Source: CAD feature listing. Evaluate the final solid. Frame: model axes, mm. A direction names the side the tool comes from. Give positions to 0.01 mm unless a question says otherwise; leave off trailing zeros. Loops run counter-clockwise (first coordinate to the right, second up) from the corner with the lowest first, then second, coordinate; pieces in that order, holes last.
```python
from build123d import *

# Parameters (mm, degrees)
F0_W     = 78
F0_H     = 157.7
F0_W_2   = 73.4
F0_H_2   = 153.1
F0_R     = 2
F0_R_2   = 2.5
F1_DEPTH = 2.3
F2_DEPTH = 9
F3_DEPTH = 7.5
F4_DEPTH = 25
F5_R     = 12
F6_R     = 14


with BuildPart() as f1:
    # F0 (on Front) → F1 (new body)
    with BuildSketch(Plane.XZ):
        Rectangle(F0_W, F0_H)
        Rectangle(F0_W_2, F0_H_2, mode=Mode.SUBTRACT)
        Rectangle(F0_W_2, F0_H_2)
        with Locations((-31.5, -22.85)):
            Circle(F0_R, mode=Mode.SUBTRACT)
        Polygon((-20, -22.85), (0, -9.85), (20, -22.85), (0, -35.85), align=None, mode=Mode.SUBTRACT)
        with Locations((31.5, -22.85)):
            Circle(F0_R, mode=Mode.SUBTRACT)
        with Locations((-30.7, 36.55)):
            Circle(F0_R, mode=Mode.SUBTRACT)
        with BuildLine():
            add(Edge.make_bspline(
                [(-20.35, 36.55), (-20.35, 29.1887840678), (-10.375, 32.8693920339), (-0.4, 36.55), (-10.375, 40.2306079661), (-20.35, 43.9112159322), (-20.35, 36.55)],
                knots=[0, 0, 0, 2.0943951024, 2.0943951024, 4.1887902048, 4.1887902048, 6.2831853072, 6.2831853072, 6.2831853072], degree=2, weights=[1, 0.5, 1, 0.5, 1, 0.5, 1]))
        make_face(mode=Mode.SUBTRACT)
        with Locations((-20.5, 60.55)):
            Circle(F0_R_2, mode=Mode.SUBTRACT)
        with BuildLine():
            ThreePointArc((2.8259154066, 10.0287804232), (1.4142570551, 10.119681178), (0, 10.15))
            ThreePointArc((0, 10.15), (-1.4142571139, 10.1196811755), (-2.825915524, 10.0287804131))
            ThreePointArc((-2.825915524, 10.0287804131), (-5.6846492436, 9.656687973), (-8.5, 9.036517527))
            Line((-8.5, 9.036517527), (0, 26.15))
            Line((0, 26.15), (8.5, 9.036517527))
            ThreePointArc((8.5, 9.036517527), (5.6846491856, 9.6566879832), (2.8259154066, 10.0287804232))
        make_face(mode=Mode.SUBTRACT)
        with BuildLine():
            add(Edge.make_bspline(
                [(20.35, 36.55), (20.35, 43.9112159322), (10.375, 40.2306079661), (0.4, 36.55), (10.375, 32.8693920339), (20.35, 29.1887840678), (20.35, 36.55)],
                knots=[0, 0, 0, 2.0943951024, 2.0943951024, 4.1887902048, 4.1887902048, 6.2831853072, 6.2831853072, 6.2831853072], degree=2, weights=[1, 0.5, 1, 0.5, 1, 0.5, 1]))
        make_face(mode=Mode.SUBTRACT)
        with Locations((30.7, 36.55)):
            Circle(F0_R, mode=Mode.SUBTRACT)
        with Locations((0, 72.05)):
            Circle(F0_R, mode=Mode.SUBTRACT)
        with Locations((20.5, 60.55)):
            Circle(F0_R_2, mode=Mode.SUBTRACT)
        Polygon((20, -22.85), (0, -9.85), (-20, -22.85), (0, -35.85), align=None)
        with BuildLine():
            ThreePointArc((-2.825915524, 10.0287804131), (-1.4142571139, 10.1196811755), (0, 10.15))
            ThreePointArc((0, 10.15), (1.4142570551, 10.119681178), (2.8259154066, 10.0287804232))
            ThreePointArc((2.8259154066, 10.0287804232), (5.6846491856, 9.6566879832), (8.5, 9.036517527))
            Line((8.5, 9.036517527), (0, 26.15))
            Line((0, 26.15), (-8.5, 9.036517527))
            ThreePointArc((-8.5, 9.036517527), (-5.6846492436, 9.656687973), (-2.825915524, 10.0287804131))
        make_face()
        with BuildLine():
            ThreePointArc((-0.54, 12.5195971139), (-1.1980972895, 10.8292141972), (-2.825915524, 10.0287804131))
            ThreePointArc((-2.825915524, 10.0287804131), (-4.8819027105, 14.2099800306), (-0.54, 12.5195971139))
        make_face(mode=Mode.SUBTRACT)
        with BuildLine():
            ThreePointArc((5.54, 12.5195971139), (4.7303828733, 10.6776943636), (2.8259154066, 10.0287804232))
            ThreePointArc((2.8259154066, 10.0287804232), (1.3496171267, 14.3614998642), (5.54, 12.5195971139))
        make_face(mode=Mode.SUBTRACT)
        with BuildLine():
            add(Edge.make_bspline(
                [(-20.35, 36.55), (-20.35, 29.1887840678), (-10.375, 32.8693920339), (-0.4, 36.55), (-10.375, 40.2306079661), (-20.35, 43.9112159322), (-20.35, 36.55)],
                knots=[0, 0, 0, 2.0943951024, 2.0943951024, 4.1887902048, 4.1887902048, 6.2831853072, 6.2831853072, 6.2831853072], degree=2, weights=[1, 0.5, 1, 0.5, 1, 0.5, 1]))
        make_face()
        with BuildLine():
            add(Edge.make_bspline(
                [(20.35, 36.55), (20.35, 43.9112159322), (10.375, 40.2306079661), (0.4, 36.55), (10.375, 32.8693920339), (20.35, 29.1887840678), (20.35, 36.55)],
                knots=[0, 0, 0, 2.0943951024, 2.0943951024, 4.1887902048, 4.1887902048, 6.2831853072, 6.2831853072, 6.2831853072], degree=2, weights=[1, 0.5, 1, 0.5, 1, 0.5, 1]))
        make_face()
        with Locations((-20.5, 60.55)):
            Circle(F0_R_2)
        with Locations((20.5, 60.55)):
            Circle(F0_R_2)
        with BuildLine():
            ThreePointArc((-0.54, 12.5195971139), (-4.8819027105, 14.2099800306), (-2.825915524, 10.0287804131))
            ThreePointArc((-2.825915524, 10.0287804131), (-1.1980972895, 10.8292141972), (-0.54, 12.5195971139))
        make_face()
        with BuildLine():
            ThreePointArc((5.54, 12.5195971139), (1.3496171267, 14.3614998642), (2.8259154066, 10.0287804232))
            ThreePointArc((2.8259154066, 10.0287804232), (4.7303828733, 10.6776943636), (5.54, 12.5195971139))
        make_face()
        with Locations((0, 72.05)):
            Circle(F0_R)
        with Locations((30.7, 36.55)):
            Circle(F0_R)
        with Locations((-30.7, 36.55)):
            Circle(F0_R)
        with Locations((-31.5, -22.85)):
            Circle(F0_R)
        with Locations((31.5, -22.85)):
            Circle(F0_R)
    extrude(amount=-F1_DEPTH)

    # F0 (on Front) → F2 (join)
    with BuildSketch(Plane.XZ):
        with Locations((-31.5, -22.85)):
            Circle(F0_R)
        with Locations((31.5, -22.85)):
            Circle(F0_R)
        with Locations((-30.7, 36.55)):
            Circle(F0_R)
        with Locations((30.7, 36.55)):
            Circle(F0_R)
        with Locations((0, 72.05)):
            Circle(F0_R)
    extrude(amount=-F2_DEPTH)

    # F0 (on Front) → F3 (cut, symmetric)
    with BuildSketch(Plane.XZ):
        with BuildLine():
            ThreePointArc((-0.54, 12.5195971139), (-4.8819027105, 14.2099800306), (-2.825915524, 10.0287804131))
            ThreePointArc((-2.825915524, 10.0287804131), (-1.1980972895, 10.8292141972), (-0.54, 12.5195971139))
        make_face()
        with BuildLine():
            ThreePointArc((5.54, 12.5195971139), (1.3496171267, 14.3614998642), (2.8259154066, 10.0287804232))
            ThreePointArc((2.8259154066, 10.0287804232), (4.7303828733, 10.6776943636), (5.54, 12.5195971139))
        make_face()
        with Locations((-20.5, 60.55)):
            Circle(F0_R_2)
        with Locations((20.5, 60.55)):
            Circle(F0_R_2)
        with BuildLine():
            add(Edge.make_bspline(
                [(-20.35, 36.55), (-20.35, 29.1887840678), (-10.375, 32.8693920339), (-0.4, 36.55), (-10.375, 40.2306079661), (-20.35, 43.9112159322), (-20.35, 36.55)],
                knots=[0, 0, 0, 2.0943951024, 2.0943951024, 4.1887902048, 4.1887902048, 6.2831853072, 6.2831853072, 6.2831853072], degree=2, weights=[1, 0.5, 1, 0.5, 1, 0.5, 1]))
        make_face()
        with BuildLine():
            add(Edge.make_bspline(
                [(20.35, 36.55), (20.35, 43.9112159322), (10.375, 40.2306079661), (0.4, 36.55), (10.375, 32.8693920339), (20.35, 29.1887840678), (20.35, 36.55)],
                knots=[0, 0, 0, 2.0943951024, 2.0943951024, 4.1887902048, 4.1887902048, 6.2831853072, 6.2831853072, 6.2831853072], degree=2, weights=[1, 0.5, 1, 0.5, 1, 0.5, 1]))
        make_face()
        Polygon((20, -22.85), (0, -9.85), (-20, -22.85), (0, -35.85), align=None)
    extrude(amount=F3_DEPTH, both=True, mode=Mode.SUBTRACT)

    # F0 (on Front) → F4 (join)
    with BuildSketch(Plane.XZ):
        Rectangle(F0_W, F0_H)
        Rectangle(F0_W_2, F0_H_2, mode=Mode.SUBTRACT)
    extrude(amount=-F4_DEPTH)

    # F5
    f5_edges = [f1.edges().sort_by_distance(p)[0] for p in [
        (36.7, 13.65, 76.55),
        (-36.7, 13.65, 76.55),
        (36.7, 13.65, -76.55),
        (-36.7, 13.65, -76.55),
    ]]
    fillet(f5_edges, radius=F5_R)

    # F6
    f6_edges = [f1.edges().sort_by_distance(p)[0] for p in [
        (39, 12.5, -78.85),
        (-39, 12.5, -78.85),
        (-39, 12.5, 78.85),
        (39, 12.5, 78.85),
    ]]
    fillet(f6_edges, radius=F6_R)


solid = f1.part
```
(1) Mould query, pull axis X, two halves, no side actions, for faces 4 (the flat face through (39, 12, -1)), 5 (the flat face through (-1, 2.3, 1)), 6 (the flat face through (-32, 9, -23)), 7 (the cylindrical face through (-35.01, 12.68, 74.64)). Classes: pulls with the +X half, pulls with the -X half, needs draft (parallel to the pull), parting line crosses it, or undercut.
A:
face 4: pulls with the +X half
face 5: undercut
face 6: undercut
face 7: pulls with the -X half
(2) Reachability of faces 1 (the flat face through (-9.86, 1.13, -16.26)), 2 (the flat face through (31, 9, -23)), 3 (the flat face through (-39, 12, -1)) from +Z, -Z, +X, -X, +Y, -Y: full face, straight path, thin tool, end or side. Return the list, or none.
A:
face 1: +Y, -Y
face 2: +Y
face 3: +Z, -Z, -X, +Y, -Y
(3) Section D-D, the plane x = -8.5. Count the separate pieces of the cut face and the enclosed holes in it, then the cut area to 3 significant figures.
A:
separate pieces: 3
enclosed holes: 0
area: 421 mm2
(4) Section A-A, the plane z = -33.5. Return the cut outline in (x, y).
A:
outline: (-39, 0) - (-3.62, 0) - (-3.62, 2.3) - (-36.7, 2.3) - (-36.7, 25) - (-39, 25) - close; (3.62, 0) - (39, 0) - (39, 25) - (36.7, 25) - (36.7, 2.3) - (3.62, 2.3) - close
(5) First-contact query: pin 1 (2 mm diameter, centred on x = 29, z = 54.5, fed in from +Y); pin 2 (2 mm diameter, centred on x = -31, z = -23, fed in from +Y); pin 3 (5 mm diameter, centred on x = -29.5, y = 6.5, fed in from +Z). Flat tips, straight axial feed; report the tip coordinate or a pass-through.
A:
pin 1: stops at y = 2.3
pin 2: stops at y = 9
pin 3: stops at z = 78.71
(6) Ray query, line 1 along X through (y, z) = (20.25, 38.5); line 2 along Z through (x, y) = (24, 19.25); line 3 along Z through (x, y) = (3.04, 0.6). Return the intervals inside material, ascending.
A:
line 1: x = -39 to -36.7, 36.7 to 39
line 2: z = -78.85 to -76.55, 76.55 to 78.85
line 3: z = -78.85 to -33.87, -11.83 to 10.02, 15.02 to 78.85
(7) Section B-B, the plane y = 12.5. Return the cut outline in (x, z).
A:
outline: (-39, -64.85) arc R14 ccw to (-25, -78.85) - (25, -78.85) arc R14 ccw to (39, -64.85) - (39, 64.85) arc R14 ccw to (25, 78.85) - (-25, 78.85) arc R14 ccw to (-39, 64.85) - close; hole (-36.7, -64.55) arc R12 ccw to (-24.7, -76.55) - (24.7, -76.55) arc R12 ccw to (36.7, -64.55) - (36.7, 64.55) arc R12 ccw to (24.7, 76.55) - (-24.7, 76.55) arc R12 ccw to (-36.7, 64.55) - close
(8) Section C-C, the plane z = 42.5. Return the cut outline in (x, y), then the cut area to 3 significant figures.
A:
outline: (-39, 0) - (39, 0) - (39, 25) - (36.7, 25) - (36.7, 2.3) - (-36.7, 2.3) - (-36.7, 25) - (-39, 25) - close
area: 284 mm2
